The drawing under review shows one solid part. Ordinate dimensions are in mm from its lowest x, y, z. A direction names the side the tool comes from. Round coordinates to 2 decimals unless told otherwise and drop trailing zeros. Use CSV: the item, a comma, the result in double quotes. Start each with the question number.
1) Machinability: for the marked faces 1 and 2, which of the approach directions +Z, -Z, +X, -X, +Y, -Y give a long, thin tool a straight path to every point of the face, cutting with its end or side? Answer none if there is none.
2) Wall thickness on probe 1 along X at (y, z) = (21.25, 36); probe 2 along X at (y, z) = (14.75, 41.5) (1 decimal): over which ranges is each line inside the solid? List them lowest first. Write a range as [from, to].
3) Mouldability with a two-part tool opening along Z and no side actions: class the marked faces 3, 4 and 5 as released by +Z, released by -Z, zero draft, split by the parting line, or undercut.
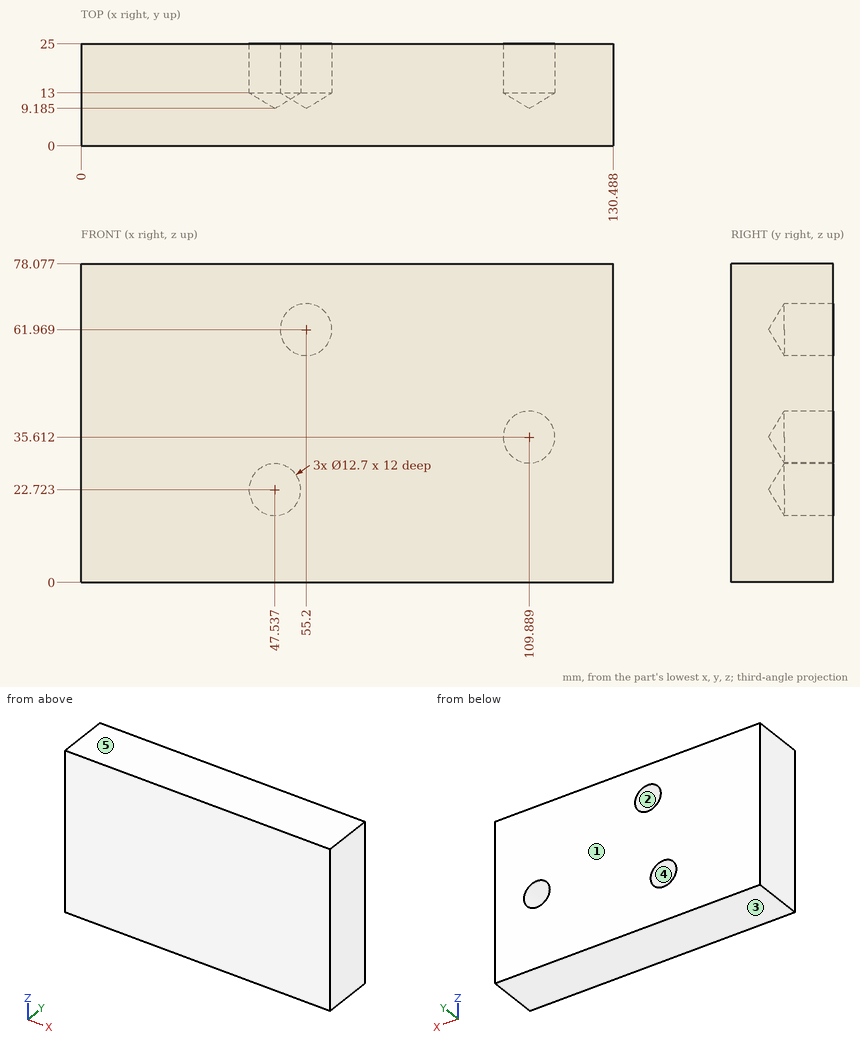
Values found:
1,face 1,"+Z, -Z, +X, -X, +Y"
1,face 2,"+Y"
2,probe 1,"[0, 103.55], [116.23, 130.49]"
2,probe 2,"[0, 107.5], [112.3, 130.5]"
3,face 3,"released by -Z"
3,face 4,"undercut"
3,face 5,"released by +Z"
